Build history of the part. All positions in model axes, mm. Face numbers are marked on the shaded views. A direction names the side the tool comes from. Round coordinates to 2 decimals unless told otherwise and drop trailing zeros. Write each loop counter-clockwise with the first axis right and the second up, starting at its lowest first coordinate (ties: lowest second). Pieces come first, ordered by that corner, then holes.
from build123d import *

# Parameters (mm, degrees)
F2_W     = 69
F2_H     = 10
F3_DEPTH = 3
F4_W     = 9
F4_H     = 3.5
F5_DEPTH = 9
F6_R     = 1
F7_DEPTH = 0.25
F8_R     = 4


with BuildPart() as f3:
    # F2 (on Top) → F3 (new body)
    with BuildSketch(Plane.XY):
        Rectangle(F2_W, F2_H)
    extrude(amount=F3_DEPTH)

    # F4 (on face) → F5 (join)
    with BuildSketch(Plane.XY.offset(3)):
        with Locations((-30, 3.25)):
            Rectangle(F4_W, F4_H)
    extrude(amount=F5_DEPTH)

    # F6 (on face) → F7 (join)
    with BuildSketch(Plane.XZ.offset(-1.5)):
        with Locations((-31.5, 6)):
            Circle(F6_R)
    extrude(amount=F7_DEPTH)

    # F8
    f8_edges = [f3.edges().sort_by_distance(p)[0] for p in [
        (-25.5, 3.25, 12),
    ]]
    fillet(f8_edges, radius=F8_R)

    # F9: F3 across plane


with BuildPart() as f3_1:
    add(f3.part)
    add(f3.part.mirror(Plane.YZ))

    # F10: F3 across plane


with BuildPart() as f3_2:
    add(f3_1.part)
    add(f3_1.part.mirror(Plane.XZ))


solid = f3_2.part
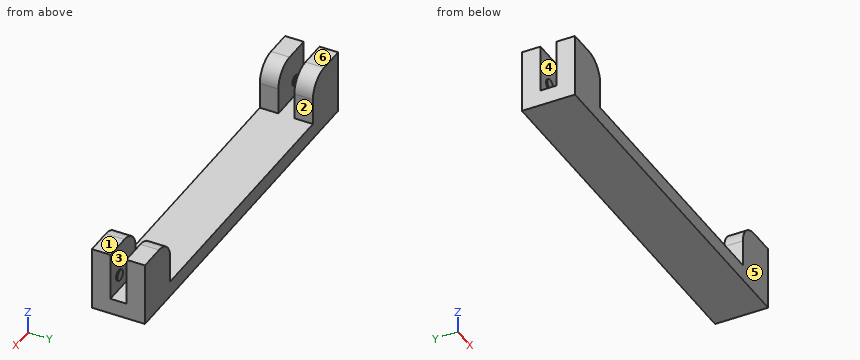
1) Mould opens along Y. For the marked faces 3, 4, 5 and 6 say: released by +Y, released by -Y, zero draft, split by the parting line, or undercut.
Results:
face 3: undercut
face 4: undercut
face 5: released by -Y
face 6: zero draft
2) Pin check, flat tip, straight feed: pin 1 Ø1.5 at (x, z) = (-6.5, 4.5) entering from +Y. Stop position of the tip, or through.
Results:
pin 1: passes through
3) Slice it at D-D (z = 8.75). Write the cut outline in (x, y), plus the area to 3 significant figures.
Results:
outline: (-34.5, -5) - (-25.57, -5) - (-25.57, -1.5) - (-34.5, -1.5) - close; (-34.5, 1.5) - (-25.57, 1.5) - (-25.57, 5) - (-34.5, 5) - close; (25.57, -5) - (34.5, -5) - (34.5, -1.5) - (25.57, -1.5) - close; (25.57, 1.5) - (34.5, 1.5) - (34.5, 5) - (25.57, 5) - close
area: 125 mm2
4) Slice it at A-A (z = 6). Count the separate pieces of the cut face and the enclosed holes in it, plus the area to 3 significant figures.
Results:
separate pieces: 4
enclosed holes: 0
area: 128 mm2
5) Which spindle directions (+Z, -Z, +X, -X, +Y, -Y) get a long thin tool onto all of the face, cutting with end or side? Do the marked faces 1 and 2. Say none if no direction does.
Results:
face 1: +Z, +X, -X, +Y, -Y
face 2: +Z, +Y, -Y
6) Slice it at C-C (y = 2.5). Write the cut outline in (x, z).
Results:
outline: (-34.5, 0) - (34.5, 0) - (34.5, 12) - (29.5, 12) arc R4 ccw to (25.5, 8) - (25.5, 3) - (-25.5, 3) - (-25.5, 8) arc R4 ccw to (-29.5, 12) - (-34.5, 12) - close
7) Slice it at B-B (x = -31.5). Write the cut outline in (y, z), plus the area to 3 significant figures.
Results:
outline: (-5, 0) - (5, 0) - (5, 12) - (1.5, 12) - (1.5, 7) - (1.25, 7) - (1.25, 5) - (1.5, 5) - (1.5, 3) - (-1.5, 3) - (-1.5, 5) - (-1.25, 5) - (-1.25, 7) - (-1.5, 7) - (-1.5, 12) - (-5, 12) - close
area: 94.0 mm2
8) Wall check: L1, parallel to X at y = 3.5, z = 6.5; L2, parallel to Y at x = 30, z = 11.75; L3, parallel to Z at x = 20, y = 4.5. Give the ranges that are in metal, low to high.
Results:
L1: x = -34.5 to -25.5, 25.5 to 34.5
L2: y = -5 to -1.5, 1.5 to 5
L3: z = 0 to 3
